CAD build for the part. Positions are in the model's coordinates, mm. A direction names the side the tool comes from. Give positions to 0.01 mm unless a question says otherwise; leave off trailing zeros. Order: outer loops, then holes, each group sorted by start corner. A loop starts at its lowest first (then second) coordinate and runs counter-clockwise, first axis right, second up. Notation, with made-up numbers: M -0.75,8 L 30.25,8 A33 cw 30.25,39 Z; hole C 31,0.25 d4. An arc over 180 degrees is marked long. Put each result on its own line as item: value. Start each with the question number.
1) Cut at D-D (y = 5.5). Write the cut outline in (x, z).
2) Cut at B-B (x = -8). Write the cut outline in (y, z).
3) Two-plate mould, pull along Y, no slides. Class faces 1 (the face through (-9, 2, 16)), 2 (the face through (-12.028, -6.595, -16.928)), 3 (the face through (-11.97, 3.4, 24.43)): released by +Y, released by -Y, zero draft, split by the parting line, or undercut.
4) Cut at C-C (z = 0). Write the cut outline in (x, y), and give its area (3 significant figures).
5) Cut at A-A (y = 32). Write the cut outline in (x, z).
6) Drill centre lines: line 1 (Y direction, x = -12.1, z = 0); line 2 (X direction, y = 1, z = -9.5); line 3 (Z direction, x = -12.5, y = 36). Where is each one in solid material? Low to high. Write a range as [from, to].
7) Tool access for faces 4 (the face through (-8, 0, -13)), 5 (the face through (-3, 20, 12)), 6 (the face through (-7, 20, 10)): list every direction of +Z, -Z, +X, -X, +Y, -Y with a clear straight run to the whole face (end or side of a thin tool).
8) Pin check, flat tips, straight feed: pin 1 (5 mm diameter, centred on x = -10, y = 29, fed in from +Z); pin 2 (2 mm diameter, centred on x = -5.5, y = 23.5, fed in from -Z); pin 3 (4 mm diameter, centred on y = -5.5, z = -15.5, fed in from +X); pin 4 (4 mm diameter, centred on y = -36.5, z = 15.5, fed in from -X). Stop position of each tip, or through.
```python
from build123d import *

# Parameters (mm, degrees)
SKETCH1_W           = 28
SKETCH1_H           = 28
SKETCH1_W_2         = 20
SKETCH1_H_2         = 20
BOSS_EXTRUDE1_DEPTH = 40
SKETCH2_R           = 2.25
CUT_EXTRUDE1_DEPTH  = 30
SKETCH5_W           = 50
SKETCH5_H           = 50
SKETCH5_R           = 1.8
SKETCH5_R_2         = 15
BOSS_EXTRUDE2_DEPTH = 4
SKETCH6_W           = 17
SKETCH6_H           = 28
CUT_EXTRUDE2_DEPTH  = 40
FILLET1_R           = 2
FILLET2_R           = 5


with BuildPart() as part:
    # Sketch1 → Boss-Extrude1 (new body)
    with BuildSketch(Plane(origin=(0, 0, 0), x_dir=(1, 0, 0), z_dir=(0, 1, 0))):
        Rectangle(SKETCH1_W, SKETCH1_H)
        Rectangle(SKETCH1_W_2, SKETCH1_H_2, mode=Mode.SUBTRACT)
    extrude(amount=BOSS_EXTRUDE1_DEPTH)

    # Sketch2 → Cut-Extrude1 (cut)
    with BuildSketch(Plane.ZY.offset(14)):
        with Locations((0, 32)):
            Circle(SKETCH2_R)
        with Locations((0, 16)):
            Circle(SKETCH2_R)
    extrude(amount=-CUT_EXTRUDE1_DEPTH, mode=Mode.SUBTRACT)

    # Sketch5 → Boss-Extrude2 (add)
    with BuildSketch(Plane.ZY.offset(14)):
        with Locations((0, -21)):
            Rectangle(SKETCH5_W, SKETCH5_H)
        with Locations((-15.499780644, -5.500219356)):
            Circle(SKETCH5_R, mode=Mode.SUBTRACT)
        with Locations((15.499780644, -5.500219356)):
            Circle(SKETCH5_R, mode=Mode.SUBTRACT)
        with Locations((15.499780644, -36.499780644)):
            Circle(SKETCH5_R, mode=Mode.SUBTRACT)
        with Locations((-15.499780644, -36.499780644)):
            Circle(SKETCH5_R, mode=Mode.SUBTRACT)
        with Locations((0, -21)):
            Circle(SKETCH5_R_2, mode=Mode.SUBTRACT)
    extrude(amount=-BOSS_EXTRUDE2_DEPTH)

    # Sketch6 → Cut-Extrude2 (cut)
    with BuildSketch(Plane.XZ):
        with Locations((5.5, 0)):
            Rectangle(SKETCH6_W, SKETCH6_H)
    extrude(amount=-CUT_EXTRUDE2_DEPTH, mode=Mode.SUBTRACT)

    # Fillet1
    fillet1_edges = [part.edges().sort_by_distance(p)[0] for p in [
        (-3, 0, -12),
        (-3, 0, 12),
        (-12, 4, 25),
        (-12, -46, 25),
        (-12, -46, -25),
        (-12, 4, -25),
        (-3, 40, -12),
        (-3, 40, 12),
    ]]
    fillet(fillet1_edges, radius=FILLET1_R)

    # Fillet2
    fillet2_edges = [part.edges().sort_by_distance(p)[0] for p in [
        (-10, 2, -14),
        (-10, 2, 14),
    ]]
    fillet(fillet2_edges, radius=FILLET2_R)


solid = part.part
```
Solution:
1. outline: M -14,-14 L -3,-14 L -3,-10 L -10,-10 L -10,10 L -3,10 L -3,14 L -14,14 Z
2. outline: M 0,-15 L 4,-15 L 4,-14 L 40,-14 L 40,-10 L 0,-10 Z; M 0,10 L 40,10 L 40,14 L 4,14 L 4,15 L 0,15 Z
3. face 1: zero draft
3. face 2: undercut
3. face 3: released by +Y
4. outline: M -14,-46 L -10,-46 L -10,-36 L -14,-36 Z; M -14,-6 L -10,-6 L -10,13.75 L -14,13.75 Z; M -14,18.25 L -10,18.25 L -10,29.75 L -14,29.75 Z; M -14,34.25 L -10,34.25 L -10,40 L -14,40 Z
4. area: 188 mm²
5. outline: M -14,-14 L -3,-14 L -3,-10 L -10,-10 L -10,-2.25 L -14,-2.25 Z; M -14,2.25 L -10,2.25 L -10,10 L -3,10 L -3,14 L -14,14 Z
6. line 1: [-46, -36], [-6, 13.75], [18.25, 29.75], [34.25, 40]
6. line 2: [-14, -10]
6. line 3: [-14, 14]
7. face 4: +Z, -Z, +X, -Y
7. face 5: +Z, -Z, +X, +Y, -Y
7. face 6: +X, +Y, -Y
8. pin 1: z = 14
8. pin 2: z = -14
8. pin 3: x = -10
8. pin 4: x = -14
